Part print with two shaded views. Sizes in mm from the minimum x, y, z corner. Coordinates: 2 decimals unless noted, no trailing zeros. Loops run counter-clockwise (first coordinate to the right, second up) from the corner with the lowest first, then second, coordinate; pieces in that order, holes last. Notation, with made-up numbers: (46.5, 63) -> (55.5, 63) arc R19 ccw to (55.5, 90) -> close; hole circle Ø8 at (87.25, -7). An arc over 180 degrees is marked (long way). Return JSON: item names as keys, results as strings. Group by question number.
(1) Saw through at C-C on y = 5. Write the cut outline in (x, z), then the cut area to 3 significant figures.
(2) Probe L1, parallel to X at y = 6.5, z = 19.5; L2, parallel to Z at x = 36.5, y = 2; L3, parallel to Z at x = 20, y = 2.75. List the from-to ranges inside material, lowest first.
(3) Saw through at A-A on x = 20. Write the cut outline in (y, z), then the cut area to 3 significant figures.
(4) Saw through at B-B on z = 20. Write the cut outline in (x, y).
(5) Saw through at D-D on x = 35.5. Write the cut outline in (y, z), then the cut area to 3 significant figures.
(6) Mould opens along Z. For the marked faces 1, 2 and 3 say: pulls with the +Z half, pulls with the -Z half, needs draft (parallel to the pull), parting line crosses it, or undercut.
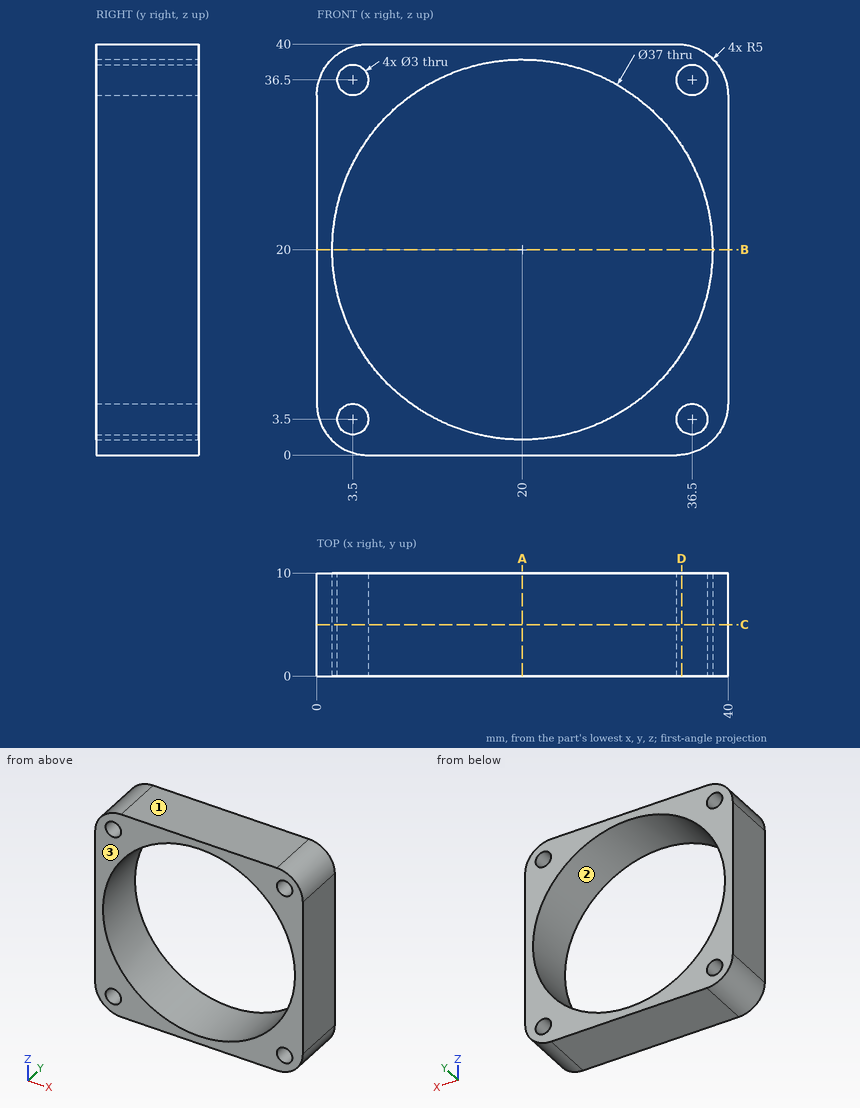
Geometry results:
{
 "1": {"outline": "(0, 5) arc R5 ccw to (5, 0) -> (35, 0) arc R5 ccw to (40, 5) -> (40, 35) arc R5 ccw to (35, 40) -> (5, 40) arc R5 ccw to (0, 35) -> close; hole circle Ø37 at (20, 20); hole circle Ø3 at (3.5, 3.5); hole circle Ø3 at (3.5, 36.5); hole circle Ø3 at (36.5, 3.5); hole circle Ø3 at (36.5, 36.5)", "area": "475 mm²"},
 "2": {"L1": "0 to 1.51, 38.49 to 40", "L2": "0.23 to 2, 5 to 11.63, 28.37 to 35, 38 to 39.77", "L3": "0 to 1.5, 38.5 to 40"},
 "3": {"outline": "(0, 0) -> (10, 0) -> (10, 1.5) -> (0, 1.5) -> close; (0, 38.5) -> (10, 38.5) -> (10, 40) -> (0, 40) -> close", "area": "30.0 mm²"},
 "4": {"outline": "(0, 0) -> (1.5, 0) -> (1.5, 10) -> (0, 10) -> close; (38.5, 0) -> (40, 0) -> (40, 10) -> (38.5, 10) -> close"},
 "5": {"outline": "(0, 0.03) -> (10, 0.03) -> (10, 2.38) -> (0, 2.38) -> close; (0, 4.62) -> (10, 4.62) -> (10, 9.9) -> (0, 9.9) -> close; (0, 30.1) -> (10, 30.1) -> (10, 35.38) -> (0, 35.38) -> close; (0, 37.62) -> (10, 37.62) -> (10, 39.97) -> (0, 39.97) -> close", "area": "153 mm²"},
 "6": {"face 1": "pulls with the +Z half", "face 2": "undercut", "face 3": "needs draft"}
}
